Build history of the part. All positions in model axes, mm. A direction names the side the tool comes from. Coordinates: 2 decimals unless noted, no trailing zeros. Loops run counter-clockwise (first coordinate to the right, second up) from the corner with the lowest first, then second, coordinate; pieces in that order, holes last. Notation, with made-up numbers: (4.5, -9) - (60.5, -9) arc R28 cw to (60.5, 11) - close; hole circle Ø8 at (89, 79). An arc over 180 degrees is marked (long way). One line per item, written item: value.
```python
from build123d import *

# Parameters (mm, degrees)
PAD016_DEPTH            = 14.9
SKETCH037_R             = 2
POCKET017_DEPTH         = 9.251
SKETCH038_R             = 3
POCKET018_DEPTH         = 2.5
BODY022_PLACEMENT_ANGLE = 180


with BuildPart() as part:
    # Sketch036 (on DatumPlane) → Pad016 (new body)
    with BuildSketch(Plane.XZ.offset(9.9)):
        with BuildLine():
            Line((-22, -0.25), (-22, -9.25))
            Line((-22, -9.25), (0, -9.25))
            Line((0, -9.25), (0, -0.25))
            Line((-6.907629, -0.25), (0, -0.25))
            ThreePointArc((-15.092371, -0.25), (-11, -4.1), (-6.907629, -0.25))
            Line((-15.092371, -0.25), (-22, -0.25))
        make_face()
    extrude(amount=PAD016_DEPTH)

    # Sketch037 → Pocket017 (cut, through all)
    with BuildSketch(Plane.XY):
        with Locations((-18.546185, -13.8)):
            Circle(SKETCH037_R)
        with Locations((-18.546185, -20.8)):
            Circle(SKETCH037_R)
        with Locations((-3.453815, -20.8)):
            Circle(SKETCH037_R)
        with Locations((-3.453815, -13.8)):
            Circle(SKETCH037_R)
    extrude(amount=-POCKET017_DEPTH, mode=Mode.SUBTRACT)

    # Sketch038 (on DatumPlane) → Pocket018 (cut)
    with BuildSketch(Plane.XY.offset(-9.25)):
        with Locations((-18.546185, -13.8)):
            Circle(SKETCH038_R)
        with Locations((-18.546185, -20.8)):
            Circle(SKETCH038_R)
        with Locations((-3.453815, -13.8)):
            Circle(SKETCH038_R)
        with Locations((-3.453815, -20.8)):
            Circle(SKETCH038_R)
    extrude(amount=POCKET018_DEPTH, mode=Mode.SUBTRACT)


with BuildPart() as part_1:
    # Body022 placement: moved
    add(part.part.moved(Location((-22, 0, -0.25))).rotate(Axis((-22, 0, -0.25), (0, 1, 0)), BODY022_PLACEMENT_ANGLE))


solid = part_1.part
```
Item 1: Cut at B-B, the plane z = 1.5. Write the cut outline in (x, y).
Check result:
outline: (-22, -24.8) - (-14.71, -24.8) - (-14.71, -9.9) - (-22, -9.9) - close; (-7.29, -24.8) - (0, -24.8) - (0, -9.9) - (-7.29, -9.9) - close; hole circle Ø4 at (-18.55, -20.8); hole circle Ø4 at (-18.55, -13.8); hole circle Ø4 at (-3.45, -20.8); hole circle Ø4 at (-3.45, -13.8)
Item 2: Cut at D-D, the plane z = 5. Write the cut outline in (x, y).
Check result:
outline: (-22, -24.8) - (0, -24.8) - (0, -9.9) - (-22, -9.9) - close; hole circle Ø4 at (-18.55, -20.8); hole circle Ø4 at (-18.55, -13.8); hole circle Ø4 at (-3.45, -20.8); hole circle Ø4 at (-3.45, -13.8)
Item 3: Cut at C-C, the plane x = -4.5. Write the cut outline in (y, z), then the cut area to 3 significant figures.
Check result:
outline: (-24.8, 0) - (-22.5, 0) - (-22.5, 6.5) - (-23.61, 6.5) - (-23.61, 9) - (-24.8, 9) - close; (-19.1, 0) - (-15.5, 0) - (-15.5, 6.5) - (-16.61, 6.5) - (-16.61, 9) - (-17.99, 9) - (-17.99, 6.5) - (-19.1, 6.5) - close; (-12.1, 0) - (-9.9, 0) - (-9.9, 9) - (-10.99, 9) - (-10.99, 6.5) - (-12.1, 6.5) - close
area: 61.7 mm^2
Item 4: Cut at A-A, the plane y = -13.8. Write the cut outline in (x, z).
Check result:
outline: (-22, 0) - (-20.55, 0) - (-20.55, 6.5) - (-21.55, 6.5) - (-21.55, 9) - (-22, 9) - close; (-16.55, 0) - (-15.09, 0) arc R4.1 cw to (-6.91, 0) - (-5.45, 0) - (-5.45, 6.5) - (-6.45, 6.5) - (-6.45, 9) - (-15.55, 9) - (-15.55, 6.5) - (-16.55, 6.5) - close; (-1.45, 0) - (0, 0) - (0, 9) - (-0.45, 9) - (-0.45, 6.5) - (-1.45, 6.5) - close
Item 5: Probe probe 1 along Y at (x, z) = (-18.5, 3.5); probe 2 along X at (y, z) = (-12.5, 1); probe 3 along X at (y, z) = (-21.25, 7.5). List the from-to ranges inside material, lowest first. Write a range as from..to.
Check result:
probe 1: y = -24.8..-22.8, -18.8..-15.8, -11.8..-9.9
probe 2: x = -22..-20.07, -17.03..-14.9, -7.1..-4.97, -1.93..0
probe 3: x = -22..-21.51, -15.58..-6.42, -0.49..0
Item 6: Drop a flat-ended pin along its axis: P1, Ø1, axis at x = -17.5, y = -19.5, coming from the +Z side. Give the stop position or say it passes through.
Check result:
P1: stops at z = 6.5
Item 7: Tool access for faces 1 (the face through (-4, -17, 0)), 2 (the face through (-18.156, -17.826, 7.768)): list every direction of +Z, -Z, +X, -X, +Y, -Y with a clear straight run to the whole face (end or side of a thin tool).
Check result:
face 1: -Z, +X, -X, +Y, -Y
face 2: +Z
Item 8: Pull direction Y, two halves, no side cores. Call faces 3 (the face through (-16.34, -11.77, 7.77)), 4 (the face through (-11, -9.9, 4)), 5 (the face through (-10.91, -17.25, 3.85)): released by +Y, released by -Y, zero draft, split by the parting line, or undercut.
Check result:
face 3: undercut
face 4: released by +Y
face 5: zero draft
